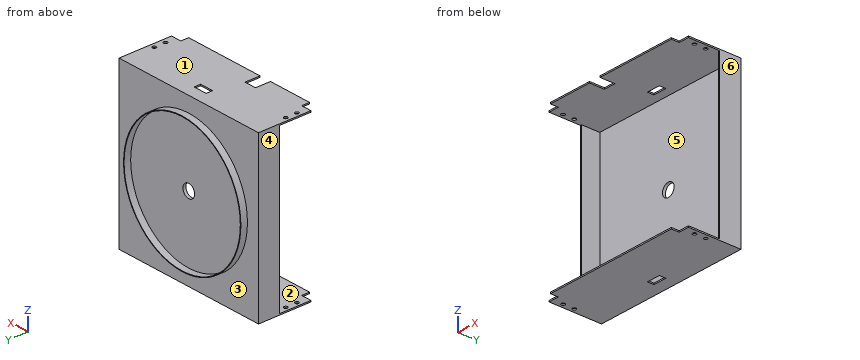
Autodesk Inventor part; units mm, degrees
ref_plane "YZ Plane" through (0, 0, 0) normal (1, 0, 0) x (0, 1, 0)
ref_plane "XZ Plane" through (0, 0, 0) normal (0, 1, 0) x (-1, 0, 0)
ref_plane "XY Plane" through (0, 0, 0) normal (0, 0, 1) x (1, 0, 0)
sketch "Sketch2" plane through (0, 0, 0) normal (0, 0, 1) x (1, 0, 0)
  line L0 (59.5, -20) -> (-59.5, -20)
  line L1 (-59.5, -20) -> (-59.5, 20)
  line L2 (-59.5, 20) -> (59.5, 20)
  line L3 (59.5, 20) -> (59.5, -20)
  line L4 (59.5, -20) -> (-59.5, 20) construction
  line L5 (-59.5, -20) -> (59.5, 20) construction
  line L6 (-59.5, -20) -> (-51.5, -20) construction
  line L7 (-51.5, -20) -> (-51.5, 4) construction
  line L8 (-51.5, 4) -> (-59.5, 4) construction
  line L9 (-59.5, 4) -> (-59.5, -20) construction
  circle A0 centre (-56.714, -3.7) radius 1.4
  circle A1 centre (-56.714, -12.2) radius 1.4
  line L10 (59.5, -20) -> (51.5, -20) construction
  line L11 (51.5, -20) -> (51.5, 4) construction
  line L12 (51.5, 4) -> (59.5, 4) construction
  line L13 (59.5, 4) -> (59.5, -20) construction
  circle A2 centre (56.4, -3.7) radius 1.4
  circle A3 centre (56.4, -12.2) radius 1.4
  line L14 (-4.7439, 11) -> (5.5561, 11)
  line L15 (5.5561, 11) -> (5.5561, 6)
  line L16 (5.5561, 6) -> (-4.7439, 6)
  line L17 (-4.7439, 6) -> (-4.7439, 11)
  line L18 (-56.714, -3.7) -> (-58.95, -3.7) construction
  point P0 (0, 0)
  dimension "d0" = 119
  dimension "d1" = 40
  dimension "d2" = 8
  dimension "d3" = 24
  dimension "d4" = 2.8
  dimension "d5" = 7.7
  dimension "d6" = 5.214
  dimension "d7" = 2.8
  dimension "d8" = 8.5
  dimension "d9" = 8
  dimension "d10" = 24
  dimension "d12" = 2.8
  dimension "d13" = 7.7
  dimension "d15" = 4.9
  dimension "d16" = 2.8
  dimension "d17" = 8.5
  dimension "d18" = 10.3
  dimension "d19" = 5
  dimension "d20" = 26
sketch "Sketch3" plane through (0, 0, 0) normal (0, 1, 0) x (-1, 0, 0)
  line L0 (-59, -61) -> (59, -61)
  line L1 (59, -61) -> (59, 61)
  line L2 (59, 61) -> (-59, 61)
  line L3 (-59, 61) -> (-59, -61)
  line L4 (-59, -61) -> (59, 61) construction
  line L5 (59, -61) -> (-59, 61) construction
  line L6 (-60, -62) -> (60, -62)
  line L7 (60, -62) -> (60, 62)
  line L8 (60, 62) -> (-60, 62)
  line L9 (-60, 62) -> (-60, -62)
  line L10 (-60, -62) -> (60, 62) construction
  line L11 (60, -62) -> (-60, 62) construction
  point P0 (0, 0)
  dimension "d21" = 118
  dimension "d22" = 122
  dimension "d23" = 120
  dimension "d24" = 124
extrude "Extrusion1" add sketch "Sketch3" along normal blind 20 and the other way blind 26 contours L3 L2 L1 L0 | L9 L8 L7 L6
extrude "Extrusion2" cut sketch "Sketch2" along normal mid plane 168.5875 contours A0 | A1 | A2 | A3 | L14 L15 L16 L17
extrude "Extrusion3" cut sketch "Sketch3" along normal blind 3.83 and the other way blind 27.3 contours L3 L2 L1 L0
sketch "Sketch4" plane through (0, 20, 0) normal (0, 1, 0) x (1, 0, 0)
  circle A0 centre (0, 0) radius 50
  circle A1 centre (0, 0) radius 50.5
  circle A2 centre (0, 0) radius 5
  dimension "d33" = 100
  dimension "d34" = 101
  dimension "d35" = 10
extrude "Extrusion4" cut sketch "Sketch4" along normal mid plane 10 contours A2
extrude "Extrusion5" add sketch "Sketch4" along normal blind 5 contours A1
sketch "Sketch5" plane through (-60, 20, 62) normal (0, 0, 1) x (1, 0, 0)
  line L0 (1, -46) -> (119, -46)
  line L1 (41.608, -46) -> (50.608, -46)
  line L2 (50.608, -46) -> (50.608, -34.6)
  line L3 (50.608, -34.6) -> (41.608, -34.6)
  line L4 (41.608, -34.6) -> (41.608, -46)
  point P0 (60, -20)
  dimension "d40" = 9
  dimension "d41" = 11.4
extrude "Extrusion6" cut sketch "Sketch5" against normal blind 5
sketch "Sketch6" plane through (60, -26, -62) normal (1, 0, 0) x (0, 0, -1)
  line L0 (-123, 0) -> (-123, 29.83)
  line L1 (-1, 0) -> (-1, 29.83)
  line L2 (-123, 29.83) -> (-1, 29.83)
  line L3 (-1, 29.83) -> (-1, 0)
  line L4 (-1, 0) -> (-123, 0)
  line L5 (-123, 0) -> (-123, 29.83)
  point P0 (-62, 26)
  point P1 (-124, 46)
extrude "Extrusion7" cut sketch "Sketch6" along normal blind 100 and the other way blind 1000
sketch "Sketch7" plane through (-60, 20, 62) normal (0, 0, 1) x (1, 0, 0)
  line L0 (0, 0) -> (0, -46) construction
  line L1 (0, 0) -> (0, -40) construction
  line L2 (0, -46) -> (0, -16.17) construction
  line L3 (0, -40) -> (8, -40) construction
  line L4 (120, -46) -> (120, 0) construction
  line L5 (120, 0) -> (120, -40) construction
  line L6 (120, -40) -> (112, -40) construction
  line L7 (112, -40) -> (112, -46) construction
  line L8 (8, -40) -> (8, -46) construction
  line L9 (0, -46) -> (120, -46) construction
  line L10 (0, -40) -> (8, -40)
  line L11 (8, -40) -> (8, -46)
  line L12 (120, -40) -> (112, -40)
  line L13 (112, -46) -> (112, -40)
  line L14 (0, -40) -> (0, -46)
  line L15 (0, -46) -> (8, -46)
  line L16 (120, -16.17) -> (120, -46)
  line L17 (120, -40) -> (120, -46)
  line L18 (120, -46) -> (112, -46)
  point P0 (60, -20)
  dimension "d55" = 40
  dimension "d56" = 8
  dimension "d57" = 40
  dimension "d58" = 8
extrude "Extrusion8" cut sketch "Sketch7" against normal blind 131.125
extrude "Extrusion9" cut sketch "Sketch3" along normal blind 17.775 contours L3 L2 L1 L0
properties part number "Upper_Housing"
CAD build for the part. Positions are in the model's coordinates, mm. Face numbers are marked on the shaded views. A direction names the side the tool comes from. Coordinates: 2 decimals unless noted, no trailing zeros. Order: outer loops, then holes, each group sorted by start corner. A loop starts at its lowest first (then second) coordinate and runs counter-clockwise, first axis right, second up. Notation, with made-up numbers: (-16, 56) - (1, 56) arc R17 cw to (1, 78) - close; hole circle Ø6 at (79, 76.5). An arc over 180 degrees is marked (long way). Answer in a Markdown table with one row per item.
1. 3-axis set-ups, long thin cutter, end or side, ignore diameter. For the marked faces 1, 2 and 3: which of +Z, -Z, +X, -X, +Y, -Y reach the whole face in a straight line?
Answer:
| item | result |
|---|---|
| face 1 | +Z, +X, -X, +Y, -Y |
| face 2 | -Y |
| face 3 | +Y |
2. Pull direction X, two halves, no side cores. Call the marked faces 4, 5 and 6: +X half, -X half, draft (parallel to the pull), parting line (faces both ways), or undercut.
Answer:
| item | result |
|---|---|
| face 4 | -X half |
| face 5 | undercut |
| face 6 | +X half |
3. Slice it at D-D, the plane x = -41. List the corners of the cut face in (y, z) (3 decimals), then the cut area to 3 significant figures.
Answer:
| item | result |
|---|---|
| outline | (-26, -62) - (20, -62) - (20, -29.483) - (25, -29.483) - (25, -28.618) - (20, -28.618) - (20, 28.618) - (25, 28.618) - (25, 29.483) - (20, 29.483) - (20, 62) - (-26, 62) - (-26, 61) - (17.775, 61) - (17.775, -61) - (-26, -61) - close |
| area | 372 mm² |
4. Flat gauge pins, fed straight in: P1, Ø0.8, axis at y = -23.5, z = 61.5, coming from the -X side; P2, Ø1.1, axis at x = 59.5, z = 2.5, coming from the -Y side; P3, Ø0.8, axis at x = 58, z = -61.5, coming from the -Y side; P4, Ø1, axis at x = 0.5, y = 9, coming from the +Z side. Where does each tip first touch, or does it go through?
Answer:
| item | result |
|---|---|
| P1 | x = -52 |
| P2 | y = 3.83 |
| P3 | y = -20 |
| P4 | through |
5. Slice it at B-B, the plane x = 0. List the corners of the cut face in (y, z) (3 decimals), then the cut area to 3 significant figures.
Answer:
| item | result |
|---|---|
| outline | (-26, -62) - (6, -62) - (6, -61) - (-26, -61) - close; (-26, 61) - (6, 61) - (6, 62) - (-26, 62) - close; (11, -62) - (20, -62) - (20, -50.5) - (25, -50.5) - (25, -50) - (20, -50) - (20, -5) - (17.775, -5) - (17.775, -61) - (11, -61) - close; (11, 61) - (17.775, 61) - (17.775, 5) - (20, 5) - (20, 50) - (25, 50) - (25, 50.5) - (20, 50.5) - (20, 62) - (11, 62) - close |
| area | 336 mm² |
6. Slice it at C-C, the plane z = 15.5. List the corners of the cut face in (x, y) (3 decimals).
Answer:
| item | result |
|---|---|
| outline | (-60, 3.83) - (-59, 3.83) - (-59, 17.775) - (59, 17.775) - (59, 3.83) - (60, 3.83) - (60, 20) - (48.062, 20) - (48.062, 25) - (47.537, 25) - (47.537, 20) - (-47.537, 20) - (-47.537, 25) - (-48.062, 25) - (-48.062, 20) - (-60, 20) - close |
7. Drill centre lines: L1, parallel to Y at x = 56.4, z = 61.55; L2, parallel to X at y = -12.2, z = 61.8; L3, parallel to Z at x = -26.5, y = -9.5. Where is each one in solid material? Low to high. Write a range as from..to.
Answer:
| item | result |
|---|---|
| L1 | -20..-13.6, -10.8..-5.1, -2.3..20 |
| L2 | -60..-58.11, -55.31..55, 57.8..60 |
| L3 | -62..-61, 61..62 |
8. Slice it at A-A, the plane z = 0. List the corners of the cut face in (x, y) (3 decimals), then the cut area to 3 significant figures.
Answer:
| item | result |
|---|---|
| outline | (-60, 3.83) - (-59, 3.83) - (-59, 17.775) - (-5, 17.775) - (-5, 20) - (-50, 20) - (-50, 25) - (-50.5, 25) - (-50.5, 20) - (-60, 20) - close; (5, 17.775) - (59, 17.775) - (59, 3.83) - (60, 3.83) - (60, 20) - (50.5, 20) - (50.5, 25) - (50, 25) - (50, 20) - (5, 20) - close |
| area | 278 mm² |
